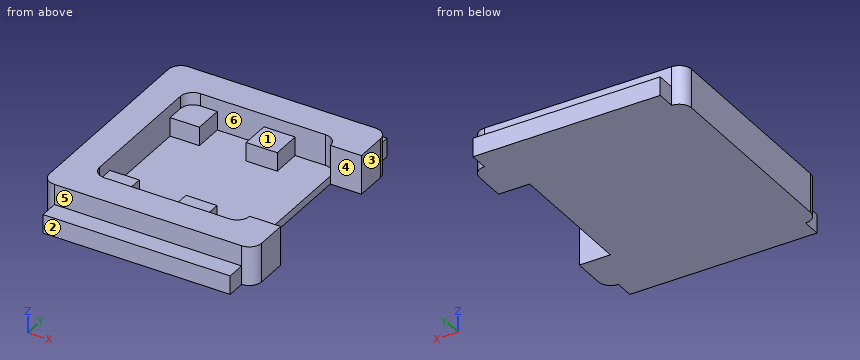
from build123d import *

# Parameters (mm, degrees)
F0_W     = 5
F0_H     = 4.7
F1_DEPTH = 1.27
F2_DEPTH = 3
F4_DEPTH = 2
F5_W     = 30.062
F5_H     = 3
F6_DEPTH = 3
F7_W     = 30.062
F7_H     = 3
F8_DEPTH = 3


with BuildPart() as f1:
    # F0 (on Top) → F1 (new body)
    with BuildSketch(Plane.XY):
        with BuildLine():
            ThreePointArc((12.031, -10.6), (11.4452135624, -12.0142135624), (10.031, -12.6))
            Line((10.031, -12.6), (5.169, -12.6))
            Line((5.169, -12.6), (0.169, -12.6))
            Line((0.169, -12.6), (-7.331, -12.6))
            Line((-7.331, -12.6), (-10.031, -12.6))
            ThreePointArc((-10.031, -12.6), (-11.4452135624, -12.0142135624), (-12.031, -10.6))
            Line((-12.031, -10.6), (-12.031, -7.9))
            Line((-12.031, -7.9), (-12.031, 7.9))
            Line((-12.031, 7.9), (-12.031, 10.6))
            ThreePointArc((-12.031, 10.6), (-11.4452135624, 12.0142135624), (-10.031, 12.6))
            Line((-10.031, 12.6), (-7.331, 12.6))
            Line((-7.331, 12.6), (0.169, 12.6))
            Line((0.169, 12.6), (5.169, 12.6))
            Line((5.169, 12.6), (10.031, 12.6))
            ThreePointArc((10.031, 12.6), (11.4452135624, 12.0142135624), (12.031, 10.6))
            Line((12.031, 10.6), (17.031, 10.6))
            Line((17.031, 10.6), (17.031, 15.6))
            ThreePointArc((17.031, 15.6), (16.4452135624, 17.0142135624), (15.031, 17.6))
            Line((15.031, 17.6), (-15.031, 17.6))
            ThreePointArc((-15.031, 17.6), (-16.4452135624, 17.0142135624), (-17.031, 15.6))
            Line((-17.031, 15.6), (-17.031, -15.6))
            ThreePointArc((-17.031, -15.6), (-16.4452135624, -17.0142135624), (-15.031, -17.6))
            Line((-15.031, -17.6), (15.031, -17.6))
            ThreePointArc((15.031, -17.6), (16.4452135624, -17.0142135624), (17.031, -15.6))
            Line((17.031, -15.6), (17.031, -10.6))
            Line((17.031, -10.6), (12.031, -10.6))
        make_face()
        with BuildLine():
            Line((5.169, -12.6), (10.031, -12.6))
            ThreePointArc((10.031, -12.6), (11.4452135624, -12.0142135624), (12.031, -10.6))
            Line((12.031, -10.6), (12.031, -10.4))
            Line((12.031, -10.4), (12.031, 10.4))
            Line((12.031, 10.4), (12.031, 10.6))
            ThreePointArc((12.031, 10.6), (11.4452135624, 12.0142135624), (10.031, 12.6))
            Line((10.031, 12.6), (5.169, 12.6))
            Line((5.169, 12.6), (5.169, 7.9))
            Line((5.169, 7.9), (0.169, 7.9))
            Line((0.169, 7.9), (0.169, 12.6))
            Line((0.169, 12.6), (-7.331, 12.6))
            Line((-7.331, 12.6), (-7.331, 7.9))
            Line((-7.331, 7.9), (-12.031, 7.9))
            Line((-12.031, 7.9), (-12.031, -7.9))
            Line((-12.031, -7.9), (-7.331, -7.9))
            Line((-7.331, -7.9), (-7.331, -12.6))
            Line((-7.331, -12.6), (0.169, -12.6))
            Line((0.169, -12.6), (0.169, -7.9))
            Line((0.169, -7.9), (5.169, -7.9))
            Line((5.169, -7.9), (5.169, -12.6))
        make_face()
        with BuildLine():
            Line((-12.031, 10.6), (-12.031, 7.9))
            Line((-12.031, 7.9), (-7.331, 7.9))
            Line((-7.331, 7.9), (-7.331, 12.6))
            Line((-7.331, 12.6), (-10.031, 12.6))
            ThreePointArc((-10.031, 12.6), (-11.4452135624, 12.0142135624), (-12.031, 10.6))
        make_face()
        with Locations((2.669, 10.25)):
            Rectangle(F0_W, F0_H)
        with Locations((2.669, -10.25)):
            Rectangle(F0_W, F0_H)
        with BuildLine():
            Line((-10.031, -12.6), (-7.331, -12.6))
            Line((-7.331, -12.6), (-7.331, -7.9))
            Line((-7.331, -7.9), (-12.031, -7.9))
            Line((-12.031, -7.9), (-12.031, -10.6))
            ThreePointArc((-12.031, -10.6), (-11.4452135624, -12.0142135624), (-10.031, -12.6))
        make_face()
    extrude(amount=-F1_DEPTH)

    # F0 (on Top) → F2 (join)
    with BuildSketch(Plane.XY):
        with BuildLine():
            ThreePointArc((12.031, -10.6), (11.4452135624, -12.0142135624), (10.031, -12.6))
            Line((10.031, -12.6), (5.169, -12.6))
            Line((5.169, -12.6), (0.169, -12.6))
            Line((0.169, -12.6), (-7.331, -12.6))
            Line((-7.331, -12.6), (-10.031, -12.6))
            ThreePointArc((-10.031, -12.6), (-11.4452135624, -12.0142135624), (-12.031, -10.6))
            Line((-12.031, -10.6), (-12.031, -7.9))
            Line((-12.031, -7.9), (-12.031, 7.9))
            Line((-12.031, 7.9), (-12.031, 10.6))
            ThreePointArc((-12.031, 10.6), (-11.4452135624, 12.0142135624), (-10.031, 12.6))
            Line((-10.031, 12.6), (-7.331, 12.6))
            Line((-7.331, 12.6), (0.169, 12.6))
            Line((0.169, 12.6), (5.169, 12.6))
            Line((5.169, 12.6), (10.031, 12.6))
            ThreePointArc((10.031, 12.6), (11.4452135624, 12.0142135624), (12.031, 10.6))
            Line((12.031, 10.6), (17.031, 10.6))
            Line((17.031, 10.6), (17.031, 15.6))
            ThreePointArc((17.031, 15.6), (16.4452135624, 17.0142135624), (15.031, 17.6))
            Line((15.031, 17.6), (-15.031, 17.6))
            ThreePointArc((-15.031, 17.6), (-16.4452135624, 17.0142135624), (-17.031, 15.6))
            Line((-17.031, 15.6), (-17.031, -15.6))
            ThreePointArc((-17.031, -15.6), (-16.4452135624, -17.0142135624), (-15.031, -17.6))
            Line((-15.031, -17.6), (15.031, -17.6))
            ThreePointArc((15.031, -17.6), (16.4452135624, -17.0142135624), (17.031, -15.6))
            Line((17.031, -15.6), (17.031, -10.6))
            Line((17.031, -10.6), (12.031, -10.6))
        make_face()
        with BuildLine():
            Line((-12.031, 10.6), (-12.031, 7.9))
            Line((-12.031, 7.9), (-7.331, 7.9))
            Line((-7.331, 7.9), (-7.331, 12.6))
            Line((-7.331, 12.6), (-10.031, 12.6))
            ThreePointArc((-10.031, 12.6), (-11.4452135624, 12.0142135624), (-12.031, 10.6))
        make_face()
        with Locations((2.669, 10.25)):
            Rectangle(F0_W, F0_H)
        with Locations((2.669, -10.25)):
            Rectangle(F0_W, F0_H)
        with BuildLine():
            Line((-10.031, -12.6), (-7.331, -12.6))
            Line((-7.331, -12.6), (-7.331, -7.9))
            Line((-7.331, -7.9), (-12.031, -7.9))
            Line((-12.031, -7.9), (-12.031, -10.6))
            ThreePointArc((-12.031, -10.6), (-11.4452135624, -12.0142135624), (-10.031, -12.6))
        make_face()
    extrude(amount=F2_DEPTH)

    # F3 (on face) → F4 (join)
    with BuildSketch(Plane.XY.offset(3)):
        with BuildLine():
            ThreePointArc((-12.031, 10.6), (-11.4452135624, 12.0142135624), (-10.031, 12.6))
            Line((-10.031, 12.6), (-7.331, 12.6))
            Line((-7.331, 12.6), (0.169, 12.6))
            Line((0.169, 12.6), (5.169, 12.6))
            Line((5.169, 12.6), (10.031, 12.6))
            ThreePointArc((10.031, 12.6), (11.4452135624, 12.0142135624), (12.031, 10.6))
            Line((12.031, 10.6), (17.031, 10.6))
            Line((17.031, 10.6), (17.031, 15.6))
            ThreePointArc((17.031, 15.6), (16.4452135624, 17.0142135624), (15.031, 17.6))
            Line((15.031, 17.6), (-15.031, 17.6))
            ThreePointArc((-15.031, 17.6), (-16.4452135624, 17.0142135624), (-17.031, 15.6))
            Line((-17.031, 15.6), (-17.031, -15.6))
            ThreePointArc((-17.031, -15.6), (-16.4452135624, -17.0142135624), (-15.031, -17.6))
            Line((-15.031, -17.6), (15.031, -17.6))
            ThreePointArc((15.031, -17.6), (16.4452135624, -17.0142135624), (17.031, -15.6))
            Line((17.031, -15.6), (17.031, -10.6))
            Line((17.031, -10.6), (12.031, -10.6))
            ThreePointArc((12.031, -10.6), (11.4452135624, -12.0142135624), (10.031, -12.6))
            Line((10.031, -12.6), (5.169, -12.6))
            Line((5.169, -12.6), (0.169, -12.6))
            Line((0.169, -12.6), (-7.331, -12.6))
            Line((-7.331, -12.6), (-10.031, -12.6))
            ThreePointArc((-10.031, -12.6), (-11.4452135624, -12.0142135624), (-12.031, -10.6))
            Line((-12.031, -10.6), (-12.031, -7.9))
            Line((-12.031, -7.9), (-12.031, 7.9))
            Line((-12.031, 7.9), (-12.031, 10.6))
        make_face()
    extrude(amount=F4_DEPTH)

    # F5 (on face) → F6 (join)
    with BuildSketch(Plane(origin=(0, 17.6, 0), x_dir=(-1, 0, 0), z_dir=(0, 1, 0))):
        with Locations((0, 0.23)):
            Rectangle(F5_W, F5_H)
    extrude(amount=F6_DEPTH)

    # F7 (on face) → F8 (join)
    with BuildSketch(Plane.XZ.offset(17.6)):
        with Locations((0, 0.23)):
            Rectangle(F7_W, F7_H)
    extrude(amount=F8_DEPTH)


solid = f1.part
The model under review builds one solid part; all positions refer to its coordinate system, in mm. Face numbers are marked on the shaded views. A direction names the side the tool comes from. Give positions to 0.01 mm unless a question says otherwise; leave off trailing zeros. Write each loop counter-clockwise with the first axis right and the second up, starting at its lowest first coordinate (ties: lowest second). Pieces come first, ordered by that corner, then holes. Notation, with made-up numbers: M 53.5,82 L 102.5,82 A16 ccw 102.5,91 Z; hole C 44,-32 d5. An arc over 180 degrees is marked long. One line per question, with ' | ' between items. Start each with the question number.
Item 1: Draft analysis for pull direction Y (two halves, no side actions). For the marked faces 1, 2 and 3, state which applies: released by +Y, released by -Y, zero draft, split by the parting line, or undercut.
Item 2: We need section B-B on x = 6. Write out the cut boundary in (y, z), plus the area to 3 significant figures.
Item 3: Wall thickness on line 1 (Y direction, x = 5, z = 0.5); line 2 (X direction, y = -12, z = 0.5); line 3 (Y direction, x = 5.5, z = 0.75): over which ranges is each line inside the solid? List them lowest first. Write a range as from..to.
Item 4: We need section C-C on y = -9. Write out the cut boundary in (x, z), plus the area to 3 significant figures.
Item 5: For the marked faces 4, 5 and 6, list the 3-axis set-ups (+Z, -Z, +X, -X, +Y, -Y) from which the entire face can be reached by the end or side of a thin tool; tool diameter is ignored.
Item 6: We need section D-D on x = 14. Write out the cut boundary in (y, z).
Item 7: For pin 1 (1.6 mm diameter, centred on x = 6, z = 3.5, fed in from +Y); pin 2 (1.5 mm diameter, centred on y = 19, z = -0.5, fed in from +X); pin 3 (2.5 mm diameter, centred on x = 3, y = -19.5, fed in from +Z), all flat-tipped, find the tip position at first contact; note any pin that passes through.
Results found:
1) face 1: undercut | face 2: released by -Y | face 3: zero draft
2) outline: M -20.6,-1.27 L 20.6,-1.27 L 20.6,1.73 L 17.6,1.73 L 17.6,5 L 12.6,5 L 12.6,0 L -12.6,0 L -12.6,5 L -17.6,5 L -17.6,1.73 L -20.6,1.73 Z | area: 113 mm2
3) line 1: y = -20.6..-7.9, 7.9..20.6 | line 2: x = -17.03..-7.33, 0.17..5.17, 11.46..17.03 | line 3: y = -20.6..-12.6, 12.6..20.6
4) outline: M -17.03,-1.27 L 12.03,-1.27 L 12.03,0 L 5.17,0 L 5.17,3 L 0.17,3 L 0.17,0 L -7.33,0 L -7.33,3 L -12.03,3 L -12.03,5 L -17.03,5 Z | area: 91.0 mm2
5) face 4: +Z, -Z, +X | face 5: +Z, +X, -X, -Y | face 6: +Z
6) outline: M -20.6,-1.27 L -10.6,-1.27 L -10.6,5 L -17.6,5 L -17.6,1.73 L -20.6,1.73 Z; M 10.6,-1.27 L 20.6,-1.27 L 20.6,1.73 L 17.6,1.73 L 17.6,5 L 10.6,5 Z
7) pin 1: stops at y = 17.6 | pin 2: stops at x = 15.03 | pin 3: stops at z = 1.73
